```python
from build123d import *

# Parameters (mm, degrees)
F1_DEPTH = 150
F2_T     = -12
F4_DEPTH = 150


with BuildPart() as f1:
    # F0 (on Right) → F1 (new body)
    with BuildSketch(Plane.YZ):
        Polygon((-150, -150), (150, -150), (150, 150), (0, 150), (0, 0), (-150, 0), align=None)
    extrude(amount=F1_DEPTH)

    # F2
    f2_openings = [f1.faces().sort_by_distance(p)[0] for p in [
        (75, 0, 75),
        (75, -75, 0),
        (75, -150, -75),
    ]]
    offset(amount=F2_T, openings=f2_openings)

    # F3 (on face) → F4 (join)
    with BuildSketch(Plane.YZ.offset(150)):
        Polygon((0, 0), (-150, 0), (-150, -12), (150, -12), (150, 0), align=None)
    extrude(amount=-F4_DEPTH)


solid = f1.part
```
Part model, mm, in its own coordinate system. A direction names the side the tool comes from. Coordinates: 2 decimals unless noted, no trailing zeros. Order: outer loops, then holes, each group sorted by start corner. A loop starts at its lowest first (then second) coordinate and runs counter-clockwise, first axis right, second up. Notation, with made-up numbers: (-31, 63) -> (-19, 63) arc R33 cw to (-19, 100) -> close; hole circle Ø10 at (27, 27.25). An arc over 180 degrees is marked (long way). Put each result on its own line as item: value. Start each with the question number.
(1) Band-saw the part on B-B (y = 21). Give the cut face in (x, z), then the cut area to 3 significant figures.
(2) Band-saw the part on A-A (x = 25). Give the cut face in (y, z), then the cut area to 3 significant figures.
(3) Pin check, flat tips, straight feed: pin 1 Ø1 at (x, y) = (32.5, -19) entering from +Z; pin 2 Ø1 at (x, z) = (94, -22.5) entering from -Y. Stop position of each tip, or through.
(4) Which spindle directions (+Z, -Z, +X, -X, +Y, -Y) get a long thin tool onto all of the face, cutting with end or side? Do faces 1 (the face through (76, -150, -141)), 2 (the face through (74, 138, 68)), 3 (the face through (80, 0, 142)). Say none if no direction does.
(5) Probe line 1 along Z through (x, y) = (126, 112); line 2 along X through (y, z) = (110, -27); line 3 along Z through (x, y) = (27, -121.5). List the from-to ranges inside material, lowest first. Write a range as [from, to].
(6) Band-saw the part on C-C (y = -43.5). Give the cut face in (x, z), then the cut area to 3 significant figures.
(7) Mould opens along X. For faces 4 (the face through (0, 31, -31)), 5 (the face through (74, 70, 138)), 6 (the face through (150, 31, -31)) say: pulls with the +X half, pulls with the -X half, needs draft (parallel to the pull), parting line crosses it, or undercut.
(8) Band-saw the part on D-D (z = 121). Give the cut face in (x, y), then the cut area to 3 significant figures.
Determined:
1. outline: (0, -150) -> (150, -150) -> (150, 150) -> (0, 150) -> close; hole (12, -138) -> (138, -138) -> (138, -12) -> (12, -12) -> close; hole (12, 0) -> (138, 0) -> (138, 138) -> (12, 138) -> close
1. area: 11,700 mm²
2. outline: (-150, -150) -> (150, -150) -> (150, 150) -> (0, 150) -> (0, 138) -> (138, 138) -> (138, 0) -> (-150, 0) -> (-150, -12) -> (138, -12) -> (138, -138) -> (-150, -138) -> close
2. area: 12,200 mm²
3. pin 1: stops at z = 0
3. pin 2: stops at y = 138
4. face 1: +Z, -Z, +X, -X, -Y
4. face 2: -Y
4. face 3: +Z, +X, -X, -Y
5. line 1: z = [-150, -138], [-12, 0], [138, 150]
5. line 2: x = [0, 12], [138, 150]
5. line 3: z = [-150, -138], [-12, 0]
6. outline: (0, -150) -> (150, -150) -> (150, 0) -> (0, 0) -> close; hole (12, -138) -> (138, -138) -> (138, -12) -> (12, -12) -> close
6. area: 6,620 mm²
7. face 4: pulls with the -X half
7. face 5: undercut
7. face 6: pulls with the +X half
8. outline: (0, 0) -> (12, 0) -> (12, 138) -> (138, 138) -> (138, 0) -> (150, 0) -> (150, 150) -> (0, 150) -> close
8. area: 5,110 mm²
